Can you work these out from the model? Positions are in its coordinate system, mm. A direction names the side the tool comes from. Round coordinates to 2 decimals unless told otherwise and drop trailing zeros. Order: outer loops, then holes, each group sorted by start corner. A loop starts at its lowest first (then second) coordinate and runs counter-clockwise, first axis right, second up. Notation, with made-up numbers: (81.5, 5) -> (100.5, 5) arc R19 ccw to (100.5, 40) -> close; hole circle Ø7 at (-36, 39). An arc over 180 degrees is marked (long way). One line per item, written item: value.
```python
from build123d import *

# Parameters (mm, degrees)
SKETCH_1_R      = 1.5
SKETCH_1_R_2    = 6
EXTRUDE_1_DEPTH = 3
FILLET_1_R      = 5


with BuildPart() as part:
    # 草图1 → 凸台-拉伸1 (new body)
    with BuildSketch(Plane(origin=(0, 0, 0), x_dir=(1, 0, 0), z_dir=(0, 1, 0))):
        with BuildLine():
            Line((-54, 50), (0, 50))
            Line((0, 50), (20, 30))
            Line((20, 30), (25, 30))
            Line((25, 30), (25, -30))
            Line((25, -30), (20, -30))
            Line((20, -30), (0, -50))
            Line((0, -50), (-54, -50))
            Line((-54, -50), (-60, -44))
            Line((-60, -44), (-60, -16))
            Line((-60, -16), (-54, -10))
            Line((-54, -10), (-25, -10))
            ThreePointArc((-25, -10), (-15, 0), (-25, 10))
            Line((-25, 10), (-54, 10))
            Line((-54, 10), (-60, 16))
            Line((-60, 16), (-60, 44))
            Line((-60, 44), (-54, 50))
        make_face()
        with Locations(Location((11, 9, 0), (0, 0, 270))):
            Circle(SKETCH_1_R, mode=Mode.SUBTRACT)
        with Locations(Location((11, -9, 0), (0, 0, 270))):
            Circle(SKETCH_1_R, mode=Mode.SUBTRACT)
        with Locations(Location((-44, -32, 0), (0, 0, 270))):
            Circle(SKETCH_1_R, mode=Mode.SUBTRACT)
        with Locations(Location((9.5, 29, 0), (0, 0, 270))):
            Circle(SKETCH_1_R, mode=Mode.SUBTRACT)
        with Locations(Location((0, 21, 0), (0, 0, 270))):
            Circle(SKETCH_1_R, mode=Mode.SUBTRACT)
        with Locations(Location((-9.5, 29, 0), (0, 0, 270))):
            Circle(SKETCH_1_R, mode=Mode.SUBTRACT)
        with Locations(Location((0, 37, 0), (0, 0, 270))):
            Circle(SKETCH_1_R, mode=Mode.SUBTRACT)
        with Locations(Location((-26, -32, 0), (0, 0, 270))):
            Circle(SKETCH_1_R, mode=Mode.SUBTRACT)
        with Locations(Location((0, -38.5, 0), (0, 0, 270))):
            Circle(SKETCH_1_R, mode=Mode.SUBTRACT)
        with Locations(Location((22, -9, 0), (0, 0, 270))):
            Circle(SKETCH_1_R, mode=Mode.SUBTRACT)
        with Locations(Location((22, 9, 0), (0, 0, 90))):
            Circle(SKETCH_1_R, mode=Mode.SUBTRACT)
        with Locations(Location((-8, -29, 0), (0, 0, 270))):
            Circle(SKETCH_1_R, mode=Mode.SUBTRACT)
        with Locations(Location((-21, -13, 0), (0, 0, 270))):
            Circle(SKETCH_1_R, mode=Mode.SUBTRACT)
        with Locations(Location((-52, 18, 0), (0, 0, 270))):
            Circle(SKETCH_1_R, mode=Mode.SUBTRACT)
        with Locations(Location((-32, 18, 0), (0, 0, 270))):
            Circle(SKETCH_1_R, mode=Mode.SUBTRACT)
        with Locations(Location((-25, 46, 0), (0, 0, 270))):
            Circle(SKETCH_1_R, mode=Mode.SUBTRACT)
        with Locations(Location((0, -19.5, 0), (0, 0, 270))):
            Circle(SKETCH_1_R, mode=Mode.SUBTRACT)
        with Locations(Location((-45, 46, 0), (0, 0, 270))):
            Circle(SKETCH_1_R, mode=Mode.SUBTRACT)
        with Locations(Location((8, -29, 0), (0, 0, 270))):
            Circle(SKETCH_1_R, mode=Mode.SUBTRACT)
        with Locations(Location((-25, -46, 0), (0, 0, 90))):
            Circle(SKETCH_1_R, mode=Mode.SUBTRACT)
        with Locations(Location((-45, -46, 0), (0, 0, 90))):
            Circle(SKETCH_1_R, mode=Mode.SUBTRACT)
        with Locations(Location((-16, -16, 0), (0, 0, 270))):
            Circle(SKETCH_1_R, mode=Mode.SUBTRACT)
        with Locations(Location((-16, -46, 0), (0, 0, 270))):
            Circle(SKETCH_1_R, mode=Mode.SUBTRACT)
        with Locations(Location((-16, 46, 0), (0, 0, 90))):
            Circle(SKETCH_1_R, mode=Mode.SUBTRACT)
        with Locations(Location((-16, 16, 0), (0, 0, 90))):
            Circle(SKETCH_1_R, mode=Mode.SUBTRACT)
        with Locations(Location((-5, 0, 0), (0, 0, 270))):
            Circle(SKETCH_1_R_2, mode=Mode.SUBTRACT)
        with Locations(Location((21, 25, 0), (0, 0, 270))):
            Circle(SKETCH_1_R, mode=Mode.SUBTRACT)
        with Locations(Location((21, -25, 0), (0, 0, 270))):
            Circle(SKETCH_1_R, mode=Mode.SUBTRACT)
        with BuildLine():
            Line((-50, 39), (-20, 39))
            ThreePointArc((-20, 39), (-18, 37), (-20, 35))
            Line((-20, 35), (-50, 35))
            ThreePointArc((-50, 35), (-52, 37), (-50, 39))
        make_face(mode=Mode.SUBTRACT)
        with BuildLine():
            Line((-50, 29), (-20, 29))
            ThreePointArc((-20, 29), (-18, 27), (-20, 25))
            Line((-20, 25), (-50, 25))
            ThreePointArc((-50, 25), (-52, 27), (-50, 29))
        make_face(mode=Mode.SUBTRACT)
        with BuildLine():
            Line((-50, -18), (-20, -18))
            ThreePointArc((-20, -18), (-18, -20), (-20, -22))
            Line((-20, -22), (-50, -22))
            ThreePointArc((-50, -22), (-52, -20), (-50, -18))
        make_face(mode=Mode.SUBTRACT)
    extrude(amount=EXTRUDE_1_DEPTH)

    # 圆角1
    fillet_1_edges = [part.edges().sort_by_distance(p)[0] for p in [
        (20, 1.5, -30),
        (20, 1.5, 30),
    ]]
    fillet(fillet_1_edges, radius=FILLET_1_R)


solid = part.part
```
Q1. I want a section at D-D on y = 1.1. Give the number of separate pieces and of enclosed holes in the cut face, plus the area to 3 significant figures.
Answers below:
separate pieces: 1
enclosed holes: 31
area: 6,270 mm^2
Q2. We'd pull the mould along Z, two halves only. Please class faces 4 (the face through (-44.1, 1.5, 47.2)), 5 (the face through (-35, 1, -29)), 6 (the face through (-60, 1, 30)), 7 (the face through (-57, 1, 47)): released by +Z, released by -Z, zero draft, split by the parting line, or undercut.
Answers below:
face 4: undercut
face 5: undercut
face 6: zero draft
face 7: released by +Z
Q3. On a 3-axis mill with a long thin cutter (end or side, diameter ignored), from which of +Z, -Z, +X, -X, +Y, -Y can I reach the whole of each face in a straight line? I mean faces 1 (the face through (-52, 1, -37)), 2 (the face through (-57, 1, 13)), 3 (the face through (24, 1, 30)). Say none if no direction works.
Answers below:
face 1: +Y, -Y
face 2: -X, +Y, -Y
face 3: +Z, +X, +Y, -Y
Q4. Please list where these lines run through material, in increasing order: line 1 along X through (y, z) = (1.6, -18); line 2 along Z through (x, y) = (-47.5, 2.2); line 3 along X through (y, z) = (1.85, 32).
Answers below:
line 1: -60 to -53.5, -50.5 to -33.5, -30.5 to 25
line 2: -50 to -39, -35 to -29, -25 to -10, 10 to 18, 22 to 50
line 3: -60 to -45.5, -42.5 to -27.5, -24.5 to 18
Q5. I want a section at B-B on x = -48.5. List the corners of the cut face in (y, z) for me.
Answers below:
outline: (0, -50) -> (3, -50) -> (3, -39) -> (0, -39) -> close; (0, -35) -> (3, -35) -> (3, -29) -> (0, -29) -> close; (0, -25) -> (3, -25) -> (3, -10) -> (0, -10) -> close; (0, 10) -> (3, 10) -> (3, 18) -> (0, 18) -> close; (0, 22) -> (3, 22) -> (3, 50) -> (0, 50) -> close
Q6. I want a section at A-A on z = 13. List the corners of the cut face in (x, y) for me.
Answers below:
outline: (-57, 0) -> (-22.5, 0) -> (-22.5, 3) -> (-57, 3) -> close; (-19.5, 0) -> (25, 0) -> (25, 3) -> (-19.5, 3) -> close
Q7. I want a section at C-C on x = -32. List the corners of the cut face in (y, z) for me.
Answers below:
outline: (0, -50) -> (3, -50) -> (3, -39) -> (0, -39) -> close; (0, -35) -> (3, -35) -> (3, -29) -> (0, -29) -> close; (0, -25) -> (3, -25) -> (3, -19.5) -> (0, -19.5) -> close; (0, -16.5) -> (3, -16.5) -> (3, -10) -> (0, -10) -> close; (0, 10) -> (3, 10) -> (3, 18) -> (0, 18) -> close; (0, 22) -> (3, 22) -> (3, 50) -> (0, 50) -> close
